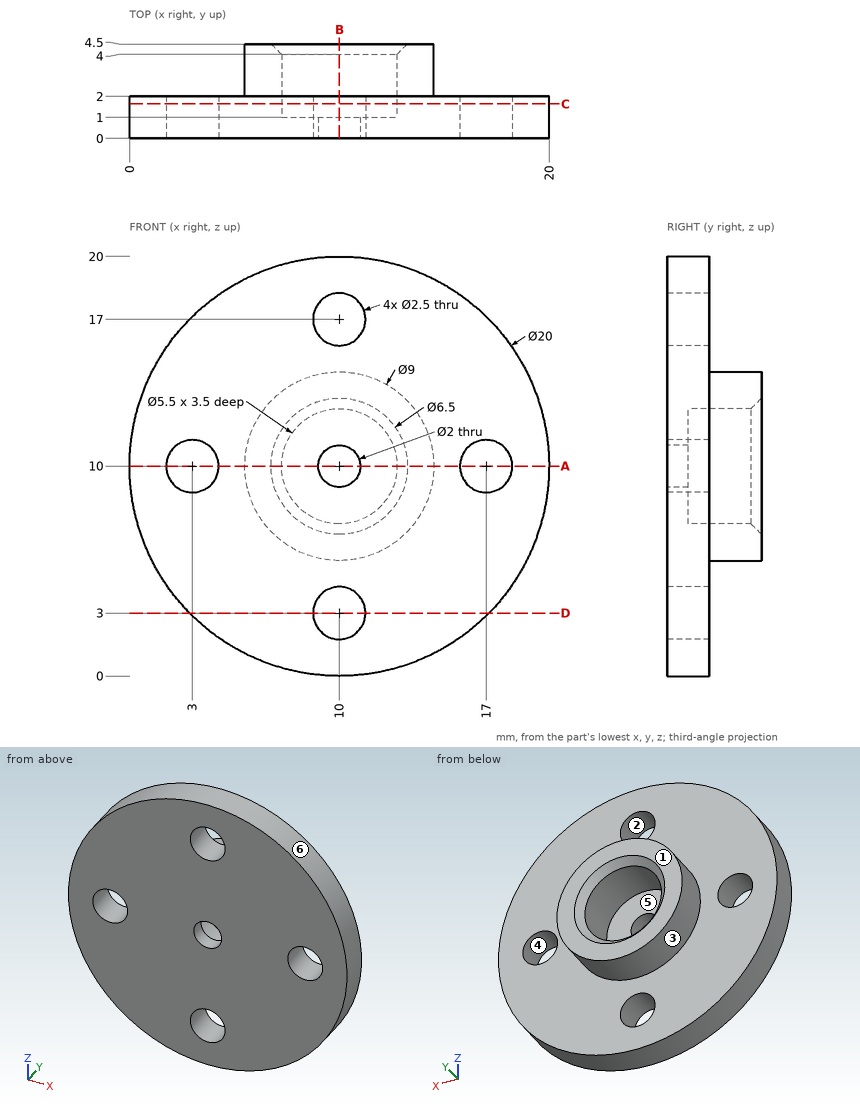
Could you check a few things on this drawing? It's one solid part, dimensions in mm from its lowest x, y, z. A direction names the side the tool comes from. Give positions to 0.01 mm unless a question says otherwise; leave off trailing zeros. Write each loop counter-clockwise with the first axis right and the second up, starting at its lowest first coordinate (ties: lowest second). Pieces come first, ordered by that corner, then holes. Notation, with made-up numbers: (-39.5, 14.25) -> (12.5, 14.25) arc R29 ccw to (12.5, 40.25) -> close; hole circle Ø1 at (18.25, 41.5). An arc over 180 degrees is marked (long way). Write each question's results on one line, items separated by ' | '.
1. I want a section at C-C, the plane y = 1.65. Write out the boundary of the cut face in (x, z).
Check sheet entries:
outline: circle Ø20 at (10, 10); hole circle Ø2.5 at (3, 10); hole circle Ø5.5 at (10, 10); hole circle Ø2.5 at (10, 3); hole circle Ø2.5 at (10, 17); hole circle Ø2.5 at (17, 10)
2. If we mould it in two halves opening along X, with no side actions, what happens to the marked faces 1, 2, 3 and 4? For each: released by +X, released by -X, zero draft, split by the parting line, or undercut.
Check sheet entries:
face 1: zero draft | face 2: undercut | face 3: split by the parting line | face 4: undercut
3. I want a section at A-A, the plane z = 10. Write out the boundary of the cut face in (x, y).
Check sheet entries:
outline: (0, 0) -> (1.75, 0) -> (1.75, 2) -> (0, 2) -> close; (4.25, 0) -> (9, 0) -> (9, 1) -> (7.25, 1) -> (7.25, 4) -> (6.75, 4.5) -> (5.5, 4.5) -> (5.5, 2) -> (4.25, 2) -> close; (11, 0) -> (15.75, 0) -> (15.75, 2) -> (14.5, 2) -> (14.5, 4.5) -> (13.25, 4.5) -> (12.75, 4) -> (12.75, 1) -> (11, 1) -> close; (18.25, 0) -> (20, 0) -> (20, 2) -> (18.25, 2) -> close
4. I want a section at D-D, the plane z = 3. Write out the boundary of the cut face in (x, y).
Check sheet entries:
outline: (2.86, 0) -> (8.75, 0) -> (8.75, 2) -> (2.86, 2) -> close; (11.25, 0) -> (17.14, 0) -> (17.14, 2) -> (11.25, 2) -> close
5. I want a section at B-B, the plane x = 10. Write out the boundary of the cut face in (y, z), then the cut area to 3 significant figures.
Check sheet entries:
outline: (0, 0) -> (2, 0) -> (2, 1.75) -> (0, 1.75) -> close; (0, 4.25) -> (2, 4.25) -> (2, 5.5) -> (4.5, 5.5) -> (4.5, 6.75) -> (4, 7.25) -> (1, 7.25) -> (1, 9) -> (0, 9) -> close; (0, 11) -> (1, 11) -> (1, 12.75) -> (4, 12.75) -> (4.5, 13.25) -> (4.5, 14.5) -> (2, 14.5) -> (2, 15.75) -> (0, 15.75) -> close; (0, 18.25) -> (2, 18.25) -> (2, 20) -> (0, 20) -> close | area: 31.0 mm²
6. On a 3-axis mill with a long thin cutter (end or side, diameter ignored), from which of +Z, -Z, +X, -X, +Y, -Y can I reach the whole of each face in a straight line? I mean the marked faces 5 and 6. Say none if no direction works.
Check sheet entries:
face 5: +Y | face 6: +Y, -Y
7. I need wall thicknesses on L1, parallel to Z at x = 10, y = 0.25; L2, parallel to Z at x = 10, y = 1.45. Which ranges of each line are inside material? Lowest first, please.
Check sheet entries:
L1: z = 0 to 1.75, 4.25 to 9, 11 to 15.75, 18.25 to 20 | L2: z = 0 to 1.75, 4.25 to 7.25, 12.75 to 15.75, 18.25 to 20
8. Will these pins go through, and if not, where does the flat tip stop? pin 1 Ø2 at (y, z) = (4, 15) entering from +X; pin 2 Ø1.5 at (y, z) = (4, 8) entering from +X.
Check sheet entries:
pin 1: stops at x = 12.06 | pin 2: stops at x = 14.32
